```python
from build123d import *

# Parameters (mm, degrees)
F0_W      = 63.5
F0_H      = 44.45
F0_W_2    = 50.292
F0_H_2    = 31.242
F1_DEPTH  = 1.5875
F2_W      = 50.292
F2_H      = 31.242
F2_W_2    = 47.117
F2_H_2    = 28.067
F3_DEPTH  = 6.35
F5_DEPTH  = 34.925
F7_DEPTH  = 38.1
F9_DEPTH  = 38.1
F11_DEPTH = 38.1
F12_R     = 3.175
F14_DEPTH = 50.292
F15_W     = 28.575
F15_H     = 4.7625
F16_DEPTH = 50.292


with BuildPart() as f1:
    # F0 (on Top) → F1 (new body)
    with BuildSketch(Plane.XY):
        Rectangle(F0_W, F0_H)
        Rectangle(F0_W_2, F0_H_2, mode=Mode.SUBTRACT)
    extrude(amount=F1_DEPTH)

    # F2 (on face) → F3 (join)
    with BuildSketch(Plane.XY.offset(1.5875)):
        Rectangle(F2_W, F2_H)
        Rectangle(F2_W_2, F2_H_2, mode=Mode.SUBTRACT)
    extrude(amount=-F3_DEPTH)

    # F4 (on Right) → F5 (join, symmetric)
    with BuildSketch(Plane.YZ):
        Polygon((-15.6114658074, 4.507067833), (0, 15.1461502537), (15.6114658074, 4.507067833), (15.6114658074, 0), (22.225, 0), (29.2133475819, -4.7625), (32.3883475819, -4.7625), (0, 17.3098860042), (-32.3883475819, -4.7625), (-29.2133475819, -4.7625), (-22.225, 0), (-15.6114658074, 0), align=None)
    extrude(amount=F5_DEPTH, both=True)

    # F6 (on Front) → F7 (cut, symmetric)
    with BuildSketch(Plane.XZ):
        Polygon((-34.925, -4.7625), (-25.4, 17.3098860042), (-34.925, 17.3098860042), align=None)
        Polygon((34.925, -4.7625), (34.925, 17.3098860042), (25.4, 17.3098860042), align=None)
    extrude(amount=F7_DEPTH, both=True, mode=Mode.SUBTRACT)

    # F8 (on Front) → F9 (join, symmetric)
    with BuildSketch(Plane.XZ):
        Polygon((-23.8125, 17.3098860042), (-25.4, 17.3098860042), (-34.925, -4.7625), (-33.3375, -4.7625), align=None)
        Polygon((34.925, -4.7625), (25.4, 17.3098860042), (23.8125, 17.3098860042), (33.3375, -4.7625), align=None)
    extrude(amount=F9_DEPTH, both=True)

    # F10 (on Right) → F11 (cut, symmetric)
    with BuildSketch(Plane.YZ):
        Polygon((-30.21584, -4.7625), (0, 17.3098860042), (-38.1, 17.3098860042), (-38.1, -4.7625), align=None)
        Polygon((38.1, 17.3098860042), (0, 17.3098860042), (30.21584, -4.7625), (38.1, -4.7625), align=None)
    extrude(amount=F11_DEPTH, both=True, mode=Mode.SUBTRACT)

    # F12
    f12_edges = [f1.edges().sort_by_distance(p)[0] for p in [
        (30.1625, -15.10792, 6.273693),
        (30.1625, 15.10792, 6.273693),
        (0, 0, 17.309886),
        (-30.1625, -15.10792, 6.273693),
        (-30.1625, 15.10792, 6.273693),
    ]]
    fillet(f12_edges, radius=F12_R)

    # F13 (on face) → F14 (join, through all)
    with BuildSketch(Plane.YZ.offset(25.146)):
        with BuildLine():
            Line((-15.621, -4.7625), (-15.621, -2.7305))
            ThreePointArc((-15.621, -2.7305), (-16.637, -3.7465), (-15.621, -4.7625))
        make_face()
        with BuildLine():
            ThreePointArc((15.621, -4.7625), (16.637, -3.7465), (15.621, -2.7305))
            Line((15.621, -2.7305), (15.621, -4.7625))
        make_face()
    extrude(amount=-F14_DEPTH)

    # F15 (on face) → F16 (cut, through all)
    with BuildSketch(Plane.YZ.offset(25.146)):
        with Locations((0, -2.38125)):
            Rectangle(F15_W, F15_H)
    extrude(amount=-F16_DEPTH, mode=Mode.SUBTRACT)


solid = f1.part
```
Geometry check sheet. Reference: the model listing, model coordinates, mm. A direction names the side the tool comes from. Coordinates: 2 decimals unless noted, no trailing zeros. One line per item, written item: value. Start each with the question number.
(1) Material ranges on line 1 (Y direction, x = 1.5, z = -1.75); line 2 (Y direction, x = -26, z = 6.25); line 3 (Y direction, x = 18, z = -3.5), recorded low to high. Write a range as [from, to].
(2) Depth check by flat-ended pin: P1, Ø8, axis at x = 17, y = -18, coming from the +Z side; P2, Ø5, axis at x = 8.5, z = 14, coming from the +Y side; P3, Ø2.5, axis at y = 16, z = -3, coming from the -X side; P4, Ø25, axis at x = -10, y = 3, coming from the +Z side. Enter the tip coordinate at first touch or a pass-through.
(3) Tool access check on faces 4 (the flat face through (-28.36, 0.22, 6.77)), 5 (the flat face through (-31.728, 0.372, 2.646)), 6 (the flat face through (23.558, 0, 1)). Record the directions out of +Z, -Z, +X, -X, +Y, -Y that give a thin tool (end or side, any length) a straight path to the whole face; none if there is none.
(4) Mould release check, pull along Z, two halves, no side actions. Record for faces 1 (the flat face through (25.146, -15, -3)), 2 (the cylindrical face through (0.352, -16.637, -3.724)), 3 (the cylindrical face through (29.88, -15.19, 5.46)): released by +Z, released by -Z, zero draft, split by the parting line, or undercut.
(5) Cross-section at B-B on z = -1. Count the separate pieces of the cut face and the enclosed holes in it, plus the area to 3 significant figures.
Results below:
1. line 1: y = [-26.09, -24.79], [-15.62, -14.29], [14.29, 15.62], [24.79, 26.09]
1. line 2: y = [-15.14, -13.05], [13.05, 15.14]
1. line 3: y = [-28.49, -27.36], [-16.61, -14.29], [14.29, 16.61], [27.36, 28.49]
2. P1: stops at z = 7.08
2. P2: stops at y = 7.95
2. P3: stops at x = -34.7
2. P4: stops at z = 16.55
3. face 4: none
3. face 5: +Z, -X, +Y, -Y
3. face 6: -Z
4. face 1: zero draft
4. face 2: undercut
4. face 3: released by +Z
5. separate pieces: 3
5. enclosed holes: 1
5. area: 461 mm2
